Design review of the part built by this model. Coordinates are the model's own, in mm. Coordinates: 2 decimals unless noted, no trailing zeros. Loops run counter-clockwise (first coordinate to the right, second up) from the corner with the lowest first, then second, coordinate; pieces in that order, holes last. Notation, with made-up numbers: (-4, 55.5) - (14, 55.5) arc R31 cw to (14, 91.5) - close; hole circle Ø5 at (8, -32.5). An arc over 180 degrees is marked (long way). One line per question, with ' | ' between items.
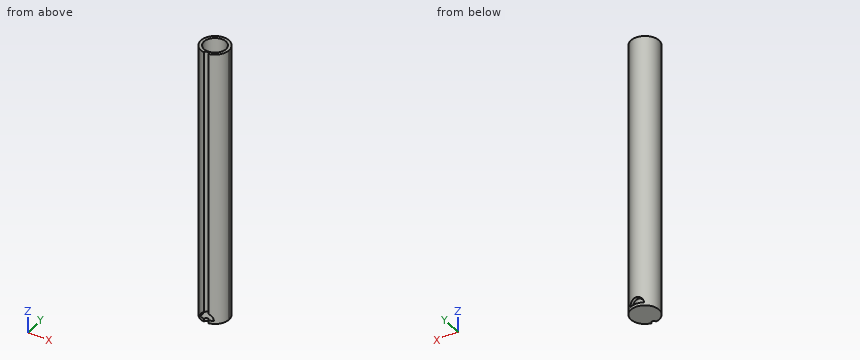
from build123d import *

# Parameters (mm, degrees)
F0_R     = 9.3
F1_DEPTH = 2
F2_R     = 9.3
F2_R_2   = 7.25
F3_DEPTH = 180
F5_DEPTH = 9.301
F6_DEPTH = 9.3010001
F8_DEPTH = 182.0010001


with BuildPart() as f1:
    # F0 (on Top) → F1 (new body)
    with BuildSketch(Plane.XY):
        Circle(F0_R)
    extrude(amount=F1_DEPTH)

    # F2 (on face) → F3 (join)
    with BuildSketch(Plane.XY.offset(2)):
        Circle(F2_R)
        Circle(F2_R_2, mode=Mode.SUBTRACT)
    extrude(amount=F3_DEPTH)

    # F4 (on Front) → F5 (cut, through all)
    with BuildSketch(Plane.XZ):
        with BuildLine():
            ThreePointArc((0, 6.4653703012), (-3.1574936205, 5.1574936205), (-4.4653703012, 2))
            Line((-4.4653703012, 2), (4.4653703012, 2))
            ThreePointArc((4.4653703012, 2), (3.1574936205, 5.1574936205), (0, 6.4653703012))
        make_face()
    extrude(amount=-F5_DEPTH, mode=Mode.SUBTRACT)

    # F4 (on Front) → F6 (cut, through all)
    with BuildSketch(Plane.XZ):
        with BuildLine():
            ThreePointArc((0, 6.4653703012), (-3.1574936205, 5.1574936205), (-4.4653703012, 2))
            Line((-4.4653703012, 2), (4.4653703012, 2))
            ThreePointArc((4.4653703012, 2), (3.1574936205, 5.1574936205), (0, 6.4653703012))
        make_face()
    extrude(amount=F6_DEPTH, mode=Mode.SUBTRACT)

    # F7 (on face) → F8 (cut, through all)
    with BuildSketch(Plane.XY.offset(182)):
        with BuildLine():
            ThreePointArc((-1.4951143118, -9.1790322581), (0, -9.3), (1.4951143118, -9.1790322581))
            ThreePointArc((1.4951143118, -9.1790322581), (0, -7.8), (-1.4951143118, -9.1790322581))
        make_face()
    extrude(amount=-F8_DEPTH, mode=Mode.SUBTRACT)


solid = f1.part
Q1. Take a section at B-B (y = -2.25). Give the boundary of the cut face in (x, z), plus the area to 3 significant figures.
Returned:
outline: (-9.02, 0) - (9.02, 0) - (9.02, 182) - (6.89, 182) - (6.89, 2) - (-6.89, 2) - (-6.89, 182) - (-9.02, 182) - close | area: 804 mm²
Q2. To check wall thickness, follow line 1 along Y through (x, z) = (0, 109); line 2 along X through (y, z) = (0, 94); line 3 along Z through (x, y) = (-2, -5.25). State the ranges of each line that lie inside material, in increasing order.
Returned:
line 1: y = -7.8 to -7.25, 7.25 to 9.3 | line 2: x = -9.3 to -7.25, 7.25 to 9.3 | line 3: z = 0 to 2
Q3. Take a section at A-A (z = 44). Give the boundary of the cut face in (x, y).
Returned:
outline: (-1.5, -9.18) arc R1.5 cw to (1.5, -9.18) arc R9.3 ccw (long way) to start; hole circle Ø14.5 at (0, 0)
Q4. For pin 1 (1 mm diameter, centred on y = 4, z = 162.5, fed in from +X); pin 2 (5 mm diameter, centred on x = -1.5, y = -0.5, fed in from +Z), all flat-tipped, find the tip position at first contact; note any pin that passes through.
Returned:
pin 1: stops at x = 8.62 | pin 2: stops at z = 2
